Input: part model. Units: mm. Frame: model coordinates. Face numbers are marked on the shaded views. Coordinates: 2 decimals unless noted, no trailing zeros. Loops run counter-clockwise (first coordinate to the right, second up) from the corner with the lowest first, then second, coordinate; pieces in that order, holes last.
Item 1: Pull-direction query (X, two-part tool) for the marked faces 1, 2 and 3; classes: released by +X, released by -X, zero draft, split by the parting line, or undercut.
Item 2: Section D-D on x = 14.5. Return loops of the section in (y, z).
Item 3: Section C-C on z = 6. Return loops of the section in (x, y), and give its area (3 significant figures).
Item 4: Section A-A on y = -1. Return loops of the section in (x, z), and give its area (3 significant figures).
Item 5: Section B-B on y = -50.5. Return loops of the section in (x, z), and give its area (3 significant figures).
Item 6: Ray query, line 1 along X through (y, z) = (-79.75, 1.4); line 2 along X through (y, z) = (-61, 6.25); line 3 along Y through (x, z) = (14.5, 2.05). Return the intervals inside material, ascending.
Item 7: Contact query for flat-ended pins moving along their axis: P1, Ø1.6, axis at x = 39.5, z = 6.5, coming from the +Y side; P2, Ø2.5, axis at y = 12, z = 9, coming from the -X side; P3, Ø6, axis at x = -12.5, z = 4, coming from the +Y side; P4, Ø3, axis at x = -5.5, z = 3, coming from the +Y side. Output: stop coordinate, or through.
```python
from build123d import *

# Parameters (mm, degrees)
PAD_DEPTH       = 3
SKETCH001_R     = 1.5
PAD001_DEPTH    = 80
SKETCH002_W     = 76
SKETCH002_H     = 10
POCKET_DEPTH    = 700
SKETCH003_R     = 2
SKETCH003_W     = 21
SKETCH003_H     = 18
POCKET001_DEPTH = 5


with BuildPart() as part:
    # Sketch → Pad (new body)
    with BuildSketch(Plane.XY):
        with BuildLine():
            Line((-40, 0), (-40, -85))
            ThreePointArc((-40, -85), (-37.803301, -90.303301), (-32.5, -92.5))
            Line((-32.5, -92.5), (32.5, -92.5))
            ThreePointArc((32.5, -92.5), (37.803301, -90.303301), (40, -85))
            Line((40, 0), (40, -85))
            Line((40, 0), (40, 17))
            Line((0, 30), (40, 17))
            Line((-40, 17), (0, 30))
            Line((-40, 0), (-40, 17))
        make_face()
    extrude(amount=PAD_DEPTH)

    # Sketch001 (on Face6 of Pad) → Pad001 (join)
    with BuildSketch(Plane.YZ.offset(40)):
        with BuildLine():
            Line((-81.5, 12), (12.5, 12))
            ThreePointArc((16, 8.5), (14.974874, 10.974874), (12.5, 12))
            Line((16, 8.5), (16, 0))
            Line((16, 0), (-85, 0))
            Line((-85, 0), (-85, 8.5))
            ThreePointArc((-81.5, 12), (-83.974874, 10.974874), (-85, 8.5))
        make_face()
        with Locations((-81, 9)):
            Circle(SKETCH001_R, mode=Mode.SUBTRACT)
        with Locations((-50.5, 9)):
            Circle(SKETCH001_R, mode=Mode.SUBTRACT)
        with Locations((-18.5, 9)):
            Circle(SKETCH001_R, mode=Mode.SUBTRACT)
        with Locations((12, 9)):
            Circle(SKETCH001_R, mode=Mode.SUBTRACT)
    extrude(amount=-PAD001_DEPTH)

    # Sketch002 (on Face7 of Pad001) → Pocket (cut)
    with BuildSketch(Plane.XZ.offset(92.5)):
        with Locations((0, 8)):
            Rectangle(SKETCH002_W, SKETCH002_H)
    extrude(amount=-POCKET_DEPTH, mode=Mode.SUBTRACT)

    # Sketch003 (on Face4 of Pocket) → Pocket001 (cut)
    with BuildSketch(Plane(origin=(0, 0, 0), x_dir=(1, 0, 0), z_dir=(0, 0, -1))):
        with Locations((14.5, 79.75)):
            Circle(SKETCH003_R)
        with Locations((-14.5, 79.75)):
            Circle(SKETCH003_R)
        with Locations((-14.5, 56.75)):
            Circle(SKETCH003_R)
        with Locations((14.5, 56.75)):
            Circle(SKETCH003_R)
        with Locations((0, 65.75)):
            Rectangle(SKETCH003_W, SKETCH003_H)
        with Locations((0, 3.25)):
            Rectangle(SKETCH003_W, SKETCH003_H)
    extrude(amount=-POCKET001_DEPTH, mode=Mode.SUBTRACT)


solid = part.part
```
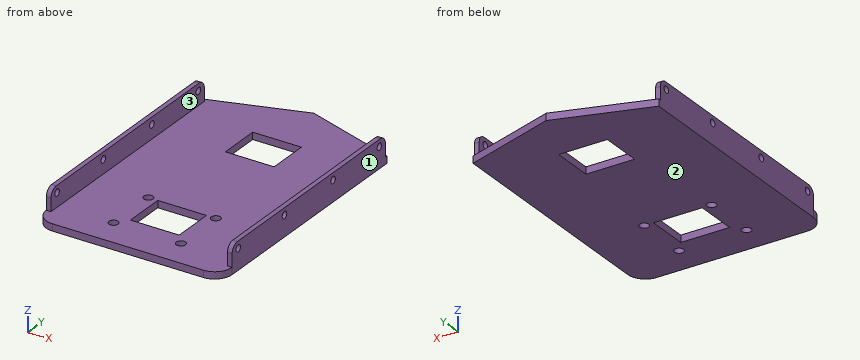
Results found:
1. face 1: released by +X
1. face 2: zero draft
1. face 3: undercut
2. outline: (-92.5, 0) - (-81.75, 0) - (-81.75, 3) - (-92.5, 3) - close; (-77.75, 0) - (-58.75, 0) - (-58.75, 3) - (-77.75, 3) - close; (-54.75, 0) - (25.29, 0) - (25.29, 3) - (-54.75, 3) - close
3. outline: (-40, -85) - (-38, -85) - (-38, 16) - (-40, 16) - close; (38, -85) - (40, -85) - (40, 16) - (38, 16) - close
3. area: 404 mm2
4. outline: (-40, 0) - (-10.5, 0) - (-10.5, 3) - (-38, 3) - (-38, 12) - (-40, 12) - close; (10.5, 0) - (40, 0) - (40, 12) - (38, 12) - (38, 3) - (10.5, 3) - close
4. area: 213 mm2
5. outline: (-40, 0) - (40, 0) - (40, 7.5) - (38, 7.5) - (38, 3) - (-38, 3) - (-38, 7.5) - (-40, 7.5) - close; (-40, 10.5) - (-38, 10.5) - (-38, 12) - (-40, 12) - close; (38, 10.5) - (40, 10.5) - (40, 12) - (38, 12) - close
5. area: 264 mm2
6. line 1: x = -40 to -16.5, -12.5 to 12.5, 16.5 to 40
6. line 2: x = -40 to -38, 38 to 40
6. line 3: y = -92.5 to -81.75, -77.75 to -58.75, -54.75 to 25.29
7. P1: stops at y = 16
7. P2: passes through
7. P3: stops at y = 26.86
7. P4: stops at y = 28.7
